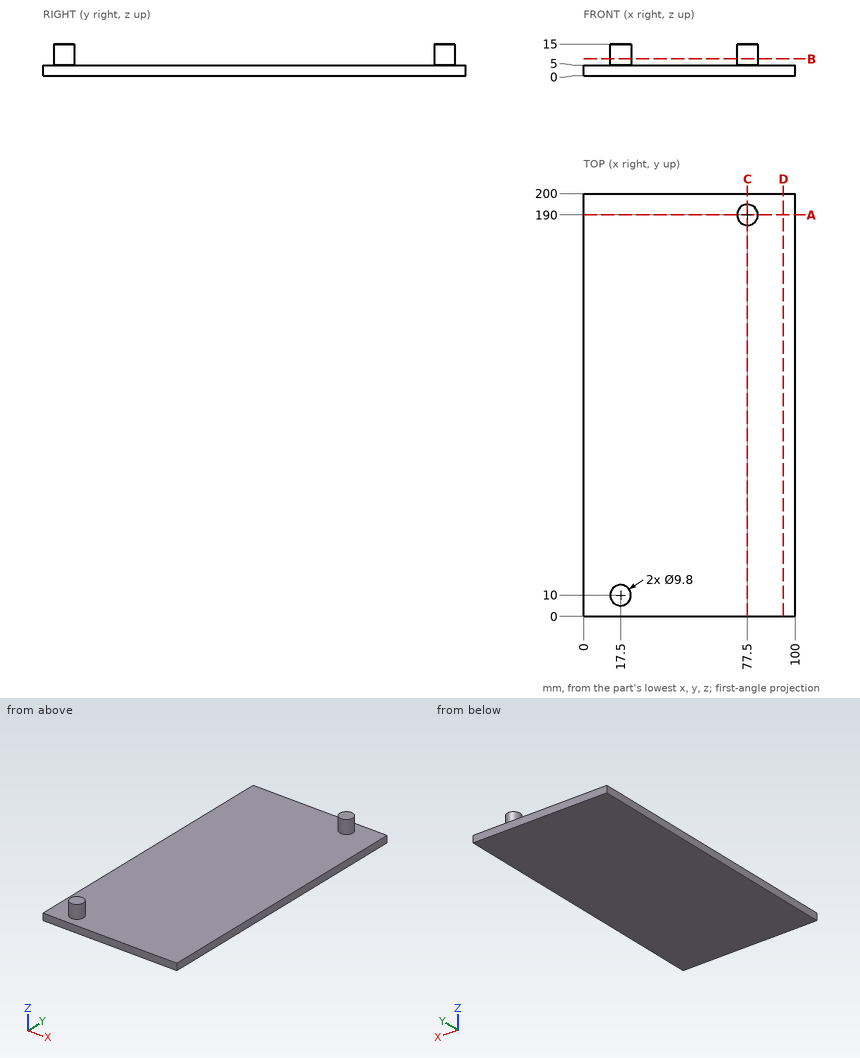
The figure shows three views and two pictorial views of one solid part (mm, origin at its lowest corner). Answer the questions. Give positions to 0.01 mm unless a question says otherwise; leave off trailing zeros. Order: outer loops, then holes, each group sorted by start corner. A loop starts at its lowest first (then second) coordinate and runs counter-clockwise, first axis right, second up. Notation, with made-up numbers: (16, 53.5) - (48, 53.5) arc R37 ccw to (48, 92.5) - close; hole circle Ø10 at (85, -28.75). An arc over 180 degrees is marked (long way). Answer as CSV lines item,"result".
Q1. Straight lines are drawn through the part: L1, parallel to Z at x = 19.5, y = 78; L2, parallel to Y at x = 18, z = 6.5; L3, parallel to Y at x = 79.5, z = 14. For each, find the intervals that lie inside material, in ascending order.
Answer key:
L1,"z = 0 to 5"
L2,"y = 5.13 to 14.87"
L3,"y = 185.53 to 194.47"
Q2. A cutting plane is placed at D-D, the plane x = 94.5. Determine the outline of the cut face in (y, z), and give its area (3 significant figures).
Answer key:
outline,"(0, 0) - (200, 0) - (200, 5) - (0, 5) - close"
area,"1,000 mm^2"
Q3. Each of these flat-tipped pins is pushed along its axis until it touches: pin 1 Ø10 at (x, y) = (42, 168.5) entering from +Z; pin 2 Ø1.5 at (y, z) = (146.5, 6) entering from -X. Where does it stop, or does it pass through?
Answer key:
pin 1,"stops at z = 5"
pin 2,"passes through"
Q4. A cutting plane is placed at A-A, the plane y = 190. Determine the outline of the cut face in (x, z), and give its area (3 significant figures).
Answer key:
outline,"(0, 0) - (100, 0) - (100, 5) - (82.4, 5) - (82.4, 15) - (72.6, 15) - (72.6, 5) - (0, 5) - close"
area,"598 mm^2"
Q5. A cutting plane is placed at C-C, the plane x = 77.5. Determine the outline of the cut face in (y, z).
Answer key:
outline,"(0, 0) - (200, 0) - (200, 5) - (194.9, 5) - (194.9, 15) - (185.1, 15) - (185.1, 5) - (0, 5) - close"
Q6. A cutting plane is placed at B-B, the plane z = 8. Determine the outline of the cut face in (x, y), and give its area (3 significant figures).
Answer key:
outline,"circle Ø9.8 at (17.5, 10); circle Ø9.8 at (77.5, 190)"
area,"151 mm^2"
